Part model, mm, in its own coordinate system. A direction names the side the tool comes from. Coordinates: 2 decimals unless noted, no trailing zeros. Write each loop counter-clockwise with the first axis right and the second up, starting at its lowest first coordinate (ties: lowest second). Pieces come first, ordered by that corner, then holes. Notation, with made-up numbers: (60, -19) -> (79, -19) arc R21 ccw to (79, -10) -> close; hole circle Ø1 at (24, -1). An arc over 180 degrees is marked (long way). One line per question, with ' | ' between items. Start each with the question number.
Item 1: Probe probe 1 along Z at (x, y) = (-3.25, 2); probe 2 along X at (y, z) = (-0.7, 1.2); probe 3 along Y at (x, z) = (-0.5, -1.85). List the from-to ranges inside material, lowest first. Write a range as [from, to].
Item 2: Two-plate mould, pull along Z, no slides. Class faces 1 (the flat face through (4.435, 0, -2)), 2 (the flat face through (1, -2, 0)), 3 (the flat face through (0, 1, -2.91)): pulls with the +Z half, pulls with the -Z half, needs draft (parallel to the pull), parting line crosses it, or undercut.
Item 3: Saw through at D-D (z = -0.05). List the corners of the cut face in (x, y).
Item 4: 3-axis set-ups, long thin cutter, end or side, ignore diameter. For faces 4 (the flat face through (-1, -2, 0)), 5 (the cylindrical face through (0.05, 0.8, 0.02)), 6 (the flat face through (0, 3.2, 2)): which of +Z, -Z, +X, -X, +Y, -Y reach the whole face in a straight line?
Item 5: Saw through at C-C (x = 0). List the corners of the cut face in (y, z).
Item 6: Pin check, flat tips, straight feed: pin 1 (1.8 mm diameter, centred on x = 0, y = -0.7, fed in from -Z); pin 2 (0.7 mm diameter, centred on y = -2.5, z = 0.5, fed in from -X); pin 3 (0.7 mm diameter, centred on y = -2.5, z = -0.5, fed in from +X). Stop position of each tip, or through.
Item 7: Saw through at B-B (z = 1.85). List the corners of the cut face in (x, y) (3 decimals).
Item 8: Saw through at A-A (y = 2). List the corners of the cut face in (x, z) (3 decimals).
Autodesk Inventor part; units mm, degrees
ref_plane "Work Plane1" through (-3.935, -0.7, 2.91) normal (0, 1, 0) x (1, 0, 0)
ref_plane "YZ Plane" through (0, 0, 0) normal (1, 0, 0) x (0, 1, 0)
ref_plane "XZ Plane" through (0, 0, 0) normal (0, 1, 0) x (-1, 0, 0)
sketch "Sketch1" plane through (0, 0, 0) normal (0, 0, 1) x (1, 0, 0)
  line L0 (-4.435, 3.2) -> (4.435, 3.2)
  line L1 (4.435, 3.2) -> (4.435, -3.2)
  line L2 (4.435, -3.2) -> (-4.435, -3.2)
  line L3 (-4.435, -3.2) -> (-4.435, 3.2)
  line L4 (0, 0) -> (4.435, 0) construction
  line L5 (0, 0) -> (0, -3.2) construction
  line L6 (0, 0) -> (0, 3.2) construction
  line L7 (0, 0) -> (-4.435, 0) construction
  dimension "d0" = 8.87
  dimension "d1" = 6.4
extrude "Extrusion1" add sketch "Sketch1" along normal mid plane 5.82
fillet "Fillet1" radius 0.5 4 edges at (4.435, -3.2, 0) (4.435, 3.2, 0) (-4.435, 3.2, 0) (-4.435, -3.2, 0)
sketch "Sketch2" plane through (0, 0, 2.91) normal (0, 0, 1) x (1, 0, 0)
  line L0 (-3.935, 3.2) -> (3.935, 3.2)
  circle A0 centre (0, -0.7) radius 1
  point P0 (0, 0)
  dimension "d5" = 3.9
  dimension "d6" = 2
extrude "Extrusion2" cut sketch "Sketch2" against normal through all
ref_plane "Work Plane1" through (-3.935, -0.7, 2.91) normal (0, 1, 0) x (1, 0, 0)
sketch "Sketch5" plane through (-3.935, -0.7, 2.91) normal (0, 1, 0) x (1, 0, 0)
  line L0 (5.435, 1.66) -> (10.1042, 1.66)
  line L1 (10.1042, 1.66) -> (10.1042, 4.16)
  line L2 (10.1042, 4.16) -> (5.435, 4.16)
  line L3 (5.435, 4.16) -> (5.435, 1.66)
  line L4 (3.935, -1.746) -> (3.935, 6.402)
  line L5 (7.87, 0) -> (0, 0)
  line L6 (0, 5.82) -> (7.87, 5.82)
  dimension "d10" = 1.5
  dimension "d11" = 1.66
  dimension "d12" = 1.66
revolve "Revolution1" cut sketch "Sketch5" angle 360 about axis through (0, -0.7, 2.91) along (0, 0, -1)
sketch "Sketch6" plane through (0, 0, 2.91) normal (0, 0, 1) x (1, 0, 0)
  circle A0 centre (0, -0.7) radius 1
  line L0 (3.935, -3.2) -> (-3.935, -3.2)
  line L1 (-1, -0.7) -> (-1, -3.2)
  line L2 (1, -0.7) -> (1, -3.2)
extrude "Extrusion3" add sketch "Sketch6" against normal through all contours L2 L0 L1 A0
properties part number "Servo Isolation Mounts1" material "ABS Plastic"
From the geometry:
1) probe 1: [-2.91, -1.25], [1.25, 2.91] | probe 2: [-1.5, -1], [1, 1.5] | probe 3: [-3.2, -1.57], [0.17, 3.2]
2) face 1: needs draft | face 2: undercut | face 3: pulls with the -Z half
3) outline: (-1, -3.2) -> (1, -3.2) -> (1, -1.82) arc R1.5 ccw (long way) to (-1, -1.82) -> close; hole circle Ø2 at (0, -0.7)
4) face 4: -X, -Y | face 5: none | face 6: +Z, -Z, +X, -X, +Y
5) outline: (-3.2, -2.91) -> (-1.7, -2.91) -> (-1.7, 2.91) -> (-3.2, 2.91) -> close; (0.3, -2.91) -> (3.2, -2.91) -> (3.2, -1.25) -> (0.8, -1.25) -> (0.8, 1.25) -> (3.2, 1.25) -> (3.2, 2.91) -> (0.3, 2.91) -> close
6) pin 1: through | pin 2: x = -1 | pin 3: x = 1
7) outline: (-4.435, -2.7) arc R0.5 ccw to (-3.935, -3.2) -> (3.935, -3.2) arc R0.5 ccw to (4.435, -2.7) -> (4.435, 2.7) arc R0.5 ccw to (3.935, 3.2) -> (-3.935, 3.2) arc R0.5 ccw to (-4.435, 2.7) -> close; hole circle Ø2 at (0, -0.7)
8) outline: (-4.435, -2.91) -> (4.435, -2.91) -> (4.435, -1.25) -> (-4.435, -1.25) -> close; (-4.435, 1.25) -> (4.435, 1.25) -> (4.435, 2.91) -> (-4.435, 2.91) -> close
